from build123d import *

# Parameters (mm, degrees)
F0_W      = 5
F0_H      = 5
F0_H_2    = 8.5
F0_W_2    = 30
F1_DEPTH  = 30
F2_DEPTH  = 2
F4_W      = 10.5
F4_H      = 30
F5_DEPTH  = 13.501
F3_R      = 5.5
F3_R_2    = 5
F3_R_3    = 2.5
F6_DEPTH  = 4
F7_DEPTH  = 5
F9_DEPTH  = 22
F10_DEPTH = 8
F11_DEPTH = 1.5
F12_R     = 5
F13_R     = 5
F15_DEPTH = 10.5
F14_R     = 2.5
F16_DEPTH = 11.5
F18_D     = 3
F20_D     = 2.5
F20_DEPTH = 15
F20_TIP   = 0.7510757738


# Not quite as in the source:
# - a feature names something its author has since deleted; it is built from what else it names


with BuildPart() as f1:
    # F0 (on Right) → F1 (new body)
    with BuildSketch(Plane.YZ):
        with Locations((17.5, 0)):
            Rectangle(F0_W, F0_H)
        with Locations((17.5, 6.75)):
            Rectangle(F0_W, F0_H_2)
        Rectangle(F0_W_2, F0_H)
        with Locations((17.5, -6.75)):
            Rectangle(F0_W, F0_H_2)
        with Locations((-17.5, 0)):
            Rectangle(F0_W, F0_H)
        with Locations((-17.5, 6.75)):
            Rectangle(F0_W, F0_H_2)
        with Locations((-17.5, -6.75)):
            Rectangle(F0_W, F0_H_2)
    extrude(amount=F1_DEPTH)

    # F0 (on Right) → F2 (join)
    with BuildSketch(Plane.YZ):
        with Locations((-17.5, 6.75)):
            Rectangle(F0_W, F0_H_2)
        with Locations((-17.5, 0)):
            Rectangle(F0_W, F0_H)
        with Locations((-17.5, -6.75)):
            Rectangle(F0_W, F0_H_2)
    extrude(amount=-F2_DEPTH)

    # F4 (on face) → F5 (cut, through all)
    with BuildSketch(Plane.XY.offset(2.5)):
        with Locations((5.25, 0)):
            Rectangle(F4_W, F4_H)
    extrude(amount=-F5_DEPTH, mode=Mode.SUBTRACT)

    # F3 (on face) → F6 (cut)
    with BuildSketch(Plane.XZ.offset(20)):
        with Locations((4.5, 0)):
            Circle(F3_R)
        with Locations((4.5, 0)):
            Circle(F3_R_2, mode=Mode.SUBTRACT)
        with Locations((4.5, 0)):
            Circle(F3_R_2)
        with Locations((4.5, 0)):
            Circle(F3_R_3, mode=Mode.SUBTRACT)
        with Locations((4.5, 0)):
            Circle(F3_R_3)
    extrude(amount=-F6_DEPTH, mode=Mode.SUBTRACT)

    # F3 (on face) → F7 (cut, through all)
    with BuildSketch(Plane.XZ.offset(20)):
        with Locations((4.5, 0)):
            Circle(F3_R_2)
        with Locations((4.5, 0)):
            Circle(F3_R_3, mode=Mode.SUBTRACT)
        with Locations((4.5, 0)):
            Circle(F3_R_3)
    extrude(amount=-F7_DEPTH, mode=Mode.SUBTRACT)

    # F8 (on face) → F9 (join, through all)
    with BuildSketch(Plane.XY.offset(11)):
        Polygon((10.5, 8.5), (10.5, 15), (0, 15), (-2, 15), (-2, 8.5), align=None)
    extrude(amount=-F9_DEPTH)

    # F10 (cut): a face of the model
    f10_faces = [f1.faces().sort_by_distance(p)[0] for p in [
        (0, 17.5, 0),
    ]]
    extrude(f10_faces, amount=-F10_DEPTH, mode=Mode.SUBTRACT)

    # F11 (cut): a face of the model
    f11_faces = [f1.faces().sort_by_distance(p)[0] for p in [
        (3, 15, 0),
    ]]
    extrude(f11_faces, amount=-F11_DEPTH, mode=Mode.SUBTRACT)

    # F12
    f12_edges = [f1.edges().sort_by_distance(p)[0] for p in [
        (8, 13.5, 0),
    ]]
    fillet(f12_edges, radius=F12_R)

    # F13
    f13_edges = [f1.edges().sort_by_distance(p)[0] for p in [
        (10.5, 15, 6.75),
        (10.5, 15, -6.75),
    ]]
    fillet(f13_edges, radius=F13_R)

    # F14 (on face) → F15 (cut)
    with BuildSketch(Plane(origin=(0, 20, 0), x_dir=(-1, 0, 0), z_dir=(0, 1, 0))):
        with BuildLine():
            Line((-8, 3.5707142143), (-8, 4.2426406871))
            ThreePointArc((-8, 4.2426406871), (-10, 0), (-8, -4.2426406871))
            Line((-8, -4.2426406871), (-8, -3.5707142143))
            ThreePointArc((-8, -3.5707142143), (-9.5, 0), (-8, 3.5707142143))
        make_face()
        with BuildLine():
            ThreePointArc((-8, -4.2426406871), (-2.1547921201, -4.9749371855), (1, 0))
            ThreePointArc((1, 0), (-2.1547921201, 4.9749371855), (-8, 4.2426406871))
            Line((-8, 4.2426406871), (-8, 3.5707142143))
            ThreePointArc((-8, 3.5707142143), (-2.5635083269, 4.6097722286), (0.5, 0))
            ThreePointArc((0.5, 0), (-2.5635083269, -4.6097722286), (-8, -3.5707142143))
            Line((-8, -3.5707142143), (-8, -4.2426406871))
        make_face()
    extrude(amount=-F15_DEPTH, mode=Mode.SUBTRACT)

    # F14 (on face) → F16 (cut, through all)
    with BuildSketch(Plane(origin=(0, 20, 0), x_dir=(-1, 0, 0), z_dir=(0, 1, 0))):
        with BuildLine():
            ThreePointArc((0.5, 0), (-2.5635083269, 4.6097722286), (-8, 3.5707142143))
            Line((-8, 3.5707142143), (-8, -3.5707142143))
            ThreePointArc((-8, -3.5707142143), (-2.5635083269, -4.6097722286), (0.5, 0))
        make_face()
        with Locations((-4.5, 0)):
            Circle(F14_R, mode=Mode.SUBTRACT)
        with Locations((-4.5, 0)):
            Circle(F14_R)
        with BuildLine():
            Line((-8, -3.5707142143), (-8, 3.5707142143))
            ThreePointArc((-8, 3.5707142143), (-9.5, 0), (-8, -3.5707142143))
        make_face()
    extrude(amount=-F16_DEPTH, mode=Mode.SUBTRACT)

    # F18 (through all)
    with Locations(Plane.YZ.offset(30)):
        with Locations((-17.5, 8.5), (-17.5, -8.5), (17.5, 8.5), (17.5, -8.5)):
            Hole(F18_D / 2)

    # F20
    with Locations(Plane(origin=(0, 20, 0), x_dir=(-1, 0, 0), z_dir=(0, 1, 0))):
        with Locations((-25, 0)):
            Hole(F20_D / 2, depth=F20_DEPTH)
            with Locations((0, 0, -(F20_DEPTH + F20_TIP / 2))):  # 118° drill point
                Cone(0, F20_D / 2, F20_TIP, mode=Mode.SUBTRACT)


solid = f1.part
The listing builds one solid part. Answer for the finished solid, in the listing's coordinates (mm). A direction names the side the tool comes from. Coordinates: 2 decimals unless noted, no trailing zeros. Order: outer loops, then holes, each group sorted by start corner. A loop starts at its lowest first (then second) coordinate and runs counter-clockwise, first axis right, second up. Notation, with made-up numbers: (86, -24.75) -> (101, -24.75) arc R30 ccw to (101, 12.25) -> close; hole circle Ø7 at (80, 18). An arc over 180 degrees is marked (long way). Answer in a Markdown table with one row per item. Add a question column.
Item 1: Determine the mould class of faces 5 (the face through (6.5, 14.93, 7.57)), 6 (the face through (10.5, 9, -7)), 7 (the face through (6, -16, -5)) for opening direction X: +X half, -X half, draft (parallel to the pull), parting line (faces both ways), or undercut.
Item 2: Find section D-D (x = 12.5). Write down the section's boundary in (y, z), then the cut area to 3 significant figures.
Item 3: Each of these flat-tipped pins is pushed along its axis until it touches: P1, Ø10, axis at x = 15.5, y = 6.5, coming from the +Z side; P2, Ø2.5, axis at y = -5, z = -1, coming from the -X side; P3, Ø0.8, axis at y = 19.5, z = 6, coming from the -X side. Where does it stop, or does it pass through?
Item 4: Find section C-C (z = 8.5). Write down the section's boundary in (x, y), then the cut area to 3 significant figures.
Item 5: Find section B-B (x = 4.5). Write down the section's boundary in (y, z), then the cut area to 3 significant figures.
Item 6: Find section A-A (y = -17.5). Write down the section's boundary in (x, z), then the cut area to 3 significant figures.
Item 7: Which of the six approach directions +Z, -Z, +X, -X, +Y, -Y give full straight-line access (tool end or side, diameter ignored) to faces 1 (the face through (8, 19.3, 7.7)), 2 (the face through (12, 13.57, 6.69)), 3 (the face through (3, 9.5, -5)), 4 (the face through (23, 15, -7))?
Item 8: Find the intervals of material crossed by L1, parallel to X at y = 12.5, z = 0; L2, parallel to Z at x = 4.5, y = -15.2; L3, parallel to Y at x = 6, z = -8.75, in increasing order. Write a range as from..to.
Result set:
| question | item | result |
|---|---|---|
| 1 | face 5 | -X half |
| 1 | face 6 | +X half |
| 1 | face 7 | undercut |
| 2 | outline | (-20, -11) -> (-15, -11) -> (-15, -2.5) -> (14, -2.5) -> (14, -11) -> (20, -11) -> (20, 11) -> (14, 11) -> (14, 2.5) -> (-15, 2.5) -> (-15, 11) -> (-20, 11) -> close; hole circle Ø3 at (-17.5, -8.5); hole circle Ø3 at (-17.5, 8.5); hole circle Ø3 at (17.5, -8.5); hole circle Ø3 at (17.5, 8.5) |
| 2 | area | 359 mm² |
| 3 | P1 | stops at z = 2.5 |
| 3 | P2 | stops at x = 10.5 |
| 3 | P3 | stops at x = 8 |
| 4 | outline | (-2, -20) -> (30, -20) -> (30, -19) -> (-2, -19) -> close; (-2, -16) -> (30, -16) -> (30, -15) -> (-2, -15) -> close; (-2, 8.5) -> (10.5, 8.5) -> (10.5, 10) arc R5 cw to (15.5, 15) -> (30, 15) -> (30, 16) -> (7.33, 16) arc R5 cw to (3, 13.5) -> (-2, 13.5) -> close; (8, 19) -> (30, 19) -> (30, 20) -> (8, 20) -> close |
| 4 | area | 184 mm² |
| 5 | outline | (-20, -11) -> (-15, -11) -> (-15, -5) -> (-16, -5) -> (-16, -5.5) -> (-20, -5.5) -> close; (-20, 5.5) -> (-16, 5.5) -> (-16, 5) -> (-15, 5) -> (-15, 11) -> (-20, 11) -> close; (8.5, -11) -> (13.73, -11) -> (13.73, -5.5) -> (9.5, -5.5) -> (9.5, -5) -> (8.5, -5) -> close; (8.5, 5) -> (9.5, 5) -> (9.5, 5.5) -> (13.73, 5.5) -> (13.73, 11) -> (8.5, 11) -> close; hole circle Ø3 at (-17.5, -8.5); hole circle Ø3 at (-17.5, 8.5) |
| 5 | area | 100 mm² |
| 6 | outline | (-2, -11) -> (30, -11) -> (30, -10) -> (-2, -10) -> close; (-2, -7) -> (30, -7) -> (30, 7) -> (-2, 7) -> close; (-2, 10) -> (30, 10) -> (30, 11) -> (-2, 11) -> close; hole circle Ø11 at (4.5, 0) |
| 6 | area | 417 mm² |
| 7 | face 1 | +Z, -Z, -X, +Y |
| 7 | face 2 | +Z, +X |
| 7 | face 3 | +Y |
| 7 | face 4 | -Z, +X |
| 8 | L1 | x = -2..-1, 10..23.75, 26.25..30 |
| 8 | L2 | z = -11..-5, 5..11 |
| 8 | L3 | y = -20..-18.98, -16.02..-15, 8.5..14.5 |
